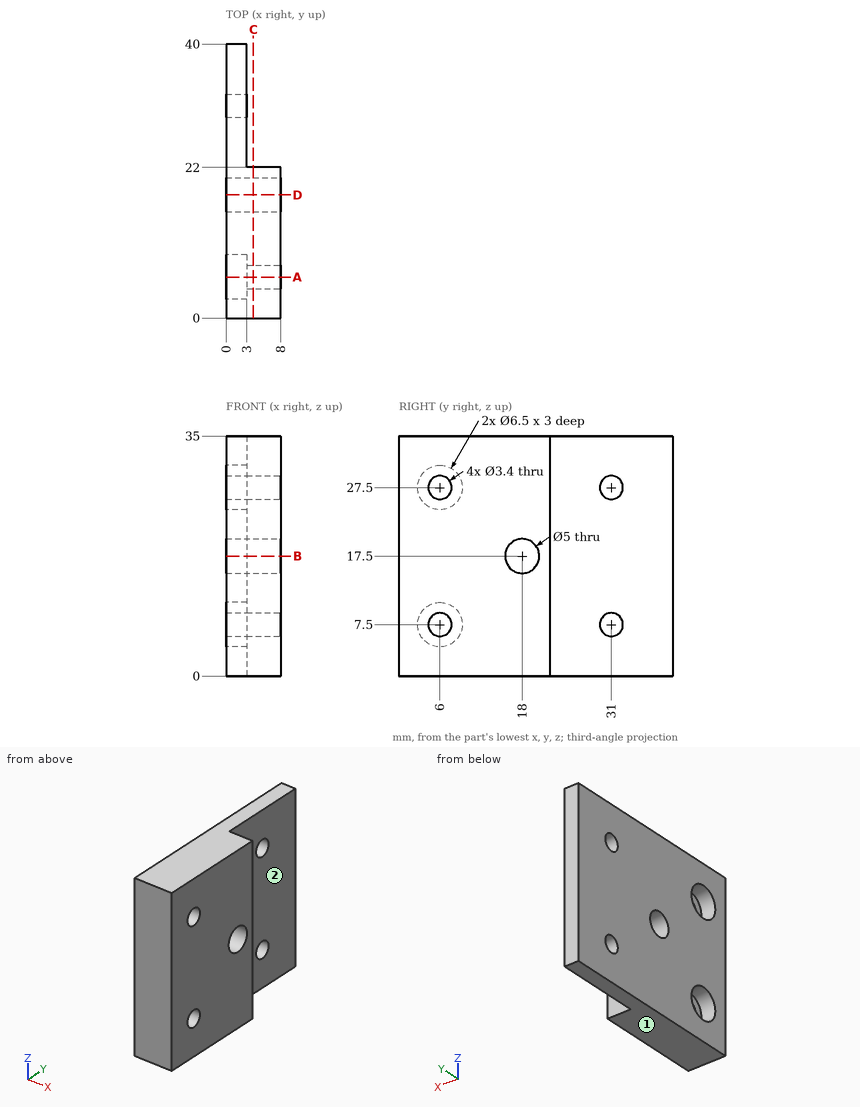
Geometry check sheet. Reference: drawing and pictorial views, mm from the part's lowest x, y, z. A direction names the side the tool comes from. Give positions to 0.01 mm unless a question says otherwise; leave off trailing zeros. Loops run counter-clockwise (first coordinate to the right, second up) from the corner with the lowest first, then second, coordinate; pieces in that order, holes last.
1. Section check A-A, the plane y = 6. Enter the section's corners in (x, z), then the cut area to 3 significant figures.
2. Section check C-C, the plane x = 4. Enter the section's corners in (y, z).
3. Section check D-D, the plane y = 18. Enter the section's corners in (x, z).
4. Thickness scan on line 1 (Y direction, x = 4.05, z = 27.5); line 2 (Y direction, x = 2.15, z = 27.5); line 3 (Y direction, x = 2.25, z = 9). Record the ranges inside material, lowest first.
5. Set-up check for the marked faces 1 and 2: record each of +Z, -Z, +X, -X, +Y, -Y from which the full face is reachable in a straight line by a thin tool's end or side.
6. Section check B-B, the plane z = 17.5. Enter the section's corners in (x, y).
7. Go/stop test with flat-tipped pins: pin 1 Ø4.5 at (y, z) = (31, 7.5) entering from +X; pin 2 Ø2 at (y, z) = (5.5, 26.5) entering from -X; pin 3 Ø2 at (x, z) = (6.5, 23.5) entering from +Y; pin 4 Ø2.5 at (y, z) = (31, 27.5) entering from -X. Record where each tip stops, or that it passes through.
Geometry says:
1. outline: (0, 0) - (8, 0) - (8, 5.8) - (3, 5.8) - (3, 4.25) - (0, 4.25) - close; (0, 10.75) - (3, 10.75) - (3, 9.2) - (8, 9.2) - (8, 25.8) - (3, 25.8) - (3, 24.25) - (0, 24.25) - close; (0, 30.75) - (3, 30.75) - (3, 29.2) - (8, 29.2) - (8, 35) - (0, 35) - close
1. area: 207 mm2
2. outline: (0, 0) - (22, 0) - (22, 35) - (0, 35) - close; hole circle Ø3.4 at (6, 7.5); hole circle Ø3.4 at (6, 27.5); hole circle Ø5 at (18, 17.5)
3. outline: (0, 0) - (8, 0) - (8, 15) - (0, 15) - close; (0, 20) - (8, 20) - (8, 35) - (0, 35) - close
4. line 1: y = 0 to 4.3, 7.7 to 22
4. line 2: y = 0 to 2.75, 9.25 to 29.3, 32.7 to 40
4. line 3: y = 0 to 3.12, 8.88 to 30.2, 31.8 to 40
5. face 1: -Z, +X, -X, +Y, -Y
5. face 2: +Z, -Z, +X, +Y
6. outline: (0, 0) - (8, 0) - (8, 15.5) - (0, 15.5) - close; (0, 20.5) - (8, 20.5) - (8, 22) - (3, 22) - (3, 40) - (0, 40) - close
7. pin 1: stops at x = 3
7. pin 2: stops at x = 3
7. pin 3: stops at y = 22
7. pin 4: passes through
